Study the drawing (mm; zero at the part's minimum x, y, z) and answer. A direction names the side the tool comes from. Round coordinates to 2 decimals unless told otherwise and drop trailing zeros. Order: outer loops, then holes, each group sorted by start corner. A loop starts at its lowest first (then second) coordinate and runs counter-clockwise, first axis right, second up. Notation, with made-up numbers: (-15, -17.5) - (5, -17.5) arc R16 cw to (5, 2.5) - close; hole circle Ø7 at (36, 83.5). An arc over 180 degrees is marked (long way). Put each result on its own line as item: value. Start each with the question number.
Q1. Section C-C on x = 79 is taken. Give the vertices of the cut face in (y, z).
Q2. For a pull along X with two mould halves and no side action, classify the marked faces 1, 2 and 3 as pulls with the +X half, pulls with the -X half, needs draft (parallel to the pull), parting line crosses it, or undercut.
Q3. Which of the six approach directions +Z, -Z, +X, -X, +Y, -Y give full straight-line access (tool end or side, diameter ignored) to the marked faces 4, 5 and 6?
Q4. Section D-D on y = 15.5 is taken. Give the vertices of the cut face in (x, z).
Q5. Find the intervals of material crossed by line 1 along X through (y, z) = (71.5, 62.5); line 2 along Y through (x, z) = (9, 57); line 3 along Y through (x, z) = (51.5, 51.5), in increasing order. Write a range as from..to.
Q6. Section A-A on y = 69 is taken. Give the vertices of the cut face in (x, z), then the cut area to 3 significant figures.
Q7. Each of these flat-tipped pins is pushed along its axis until it touches: pin 1 Ø12 at (y, z) = (70.5, 37) entering from -X; pin 2 Ø1.5 at (x, z) = (62.5, 52) entering from +Y; pin 3 Ø6 at (x, y) = (49, 66.5) entering from +Z. Where does it stop, or does it pass through?
Q8. Section B-B on z = 35 is taken. Give the vertices of the cut face in (x, y), then the cut area to 3 significant figures.
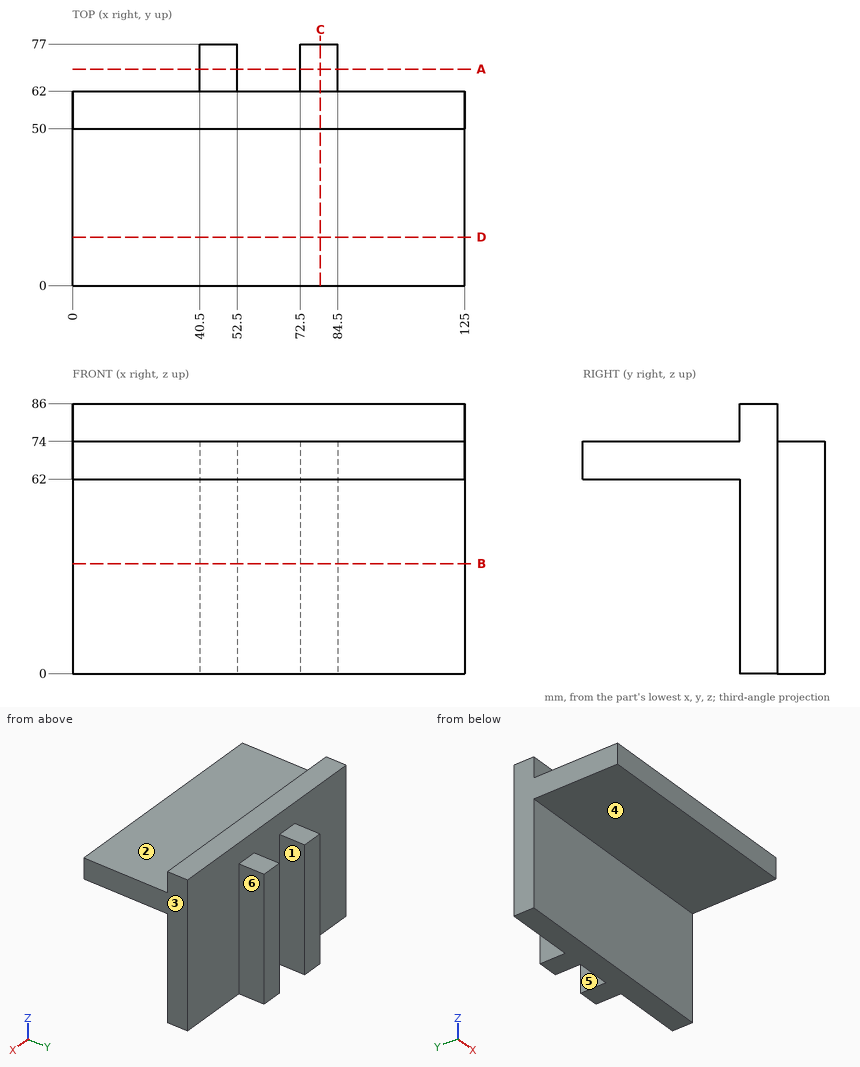
Findings:
1. outline: (0, 62) - (50, 62) - (50, 0) - (77, 0) - (77, 74) - (62, 74) - (62, 86) - (50, 86) - (50, 74) - (0, 74) - close
2. face 1: undercut
2. face 2: needs draft
2. face 3: pulls with the +X half
3. face 4: -Z, +X, -X, -Y
3. face 5: +Z, -Z, +Y
3. face 6: +Z, -Z, +X, +Y
4. outline: (0, 62) - (125, 62) - (125, 74) - (0, 74) - close
5. line 1: 40.5..52.5, 72.5..84.5
5. line 2: 50..62
5. line 3: 50..77
6. outline: (40.5, 0) - (52.5, 0) - (52.5, 74) - (40.5, 74) - close; (72.5, 0) - (84.5, 0) - (84.5, 74) - (72.5, 74) - close
6. area: 1,780 mm2
7. pin 1: x = 40.5
7. pin 2: y = 62
7. pin 3: z = 74
8. outline: (0, 50) - (125, 50) - (125, 62) - (84.5, 62) - (84.5, 77) - (72.5, 77) - (72.5, 62) - (52.5, 62) - (52.5, 77) - (40.5, 77) - (40.5, 62) - (0, 62) - close
8. area: 1,860 mm2
